Model file for the job. Use its own axes, mm. Face numbers are marked on the shaded views. A direction names the side the tool comes from. Coordinates: 2 decimals unless noted, no trailing zeros. Loops run counter-clockwise (first coordinate to the right, second up) from the corner with the lowest first, then second, coordinate; pieces in that order, holes last.
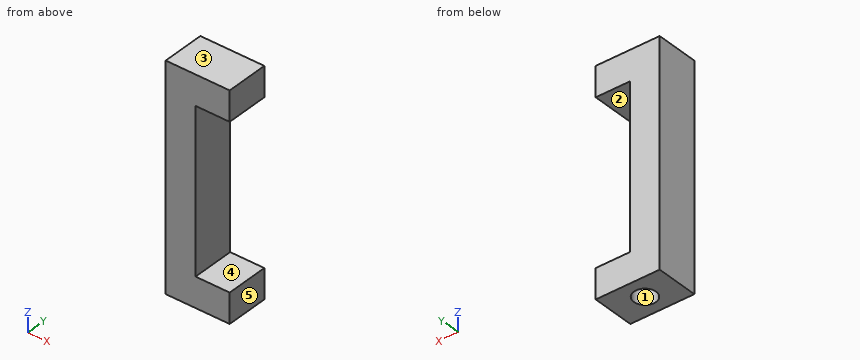
from build123d import *

# Parameters (mm, degrees)
F1_DEPTH      = 12.5
F1_DEPTH_BACK = 12.5
F2_R          = 6.5
F3_DEPTH      = 12


with BuildPart() as f1:
    # F0 (on Front) → F1 (new body, two sides)
    with BuildSketch(Plane.XZ) as f1_sk:
        Polygon((0, 65), (0, 0), (0, -65), (37.5, -65), (37.5, -47.5), (17.5, -47.5), (17.5, 0), (17.5, 47.5), (37.5, 47.5), (37.5, 65), align=None)
    extrude(amount=F1_DEPTH)
    extrude(f1_sk.sketch, amount=-F1_DEPTH_BACK)

    # F2 (on face) → F3 (cut)
    with BuildSketch(Plane(origin=(0, 0, -65), x_dir=(1, 0, 0), z_dir=(0, 0, -1))):
        with Locations((18.75, 0)):
            Circle(F2_R)
    extrude(amount=-F3_DEPTH, mode=Mode.SUBTRACT)


solid = f1.part
Q1. Slice it at A-A (x = 18.75). List the corners of the cut face in (y, z), and give its area (3 significant figures).
Answers:
outline: (-12.5, -65) - (-6.5, -65) - (-6.5, -53) - (6.5, -53) - (6.5, -65) - (12.5, -65) - (12.5, -47.5) - (-12.5, -47.5) - close; (-12.5, 47.5) - (12.5, 47.5) - (12.5, 65) - (-12.5, 65) - close
area: 719 mm2
Q2. Mould opens along Z. For the marked faces 1, 2 and 3 say: +Z half, -Z half, draft (parallel to the pull), parting line (faces both ways), or undercut.
Answers:
face 1: draft
face 2: undercut
face 3: +Z half
Q3. Slice it at C-C (x = 31). List the corners of the cut face in (y, z).
Answers:
outline: (-12.5, -65) - (12.5, -65) - (12.5, -47.5) - (-12.5, -47.5) - close; (-12.5, 47.5) - (12.5, 47.5) - (12.5, 65) - (-12.5, 65) - close
Q4. Slice it at D-D (z = -36.5). List the corners of the cut face in (x, y).
Answers:
outline: (0, -12.5) - (17.5, -12.5) - (17.5, 12.5) - (0, 12.5) - close
Q5. Slice it at B-B (y = 8). List the corners of the cut face in (x, z), and give its area (4 significant figures).
Answers:
outline: (0, -65) - (37.5, -65) - (37.5, -47.5) - (17.5, -47.5) - (17.5, 47.5) - (37.5, 47.5) - (37.5, 65) - (0, 65) - close
area: 2,975 mm2
Q6. Flat gauge pin, fed straight in: P1, Ø2, axis at y = 0, z = 36, coming from the +X side. Where does the tip first touch, or does it go through?
Answers:
P1: stops at x = 17.5
Q7. Which spindle directions (+Z, -Z, +X, -X, +Y, -Y) get a long thin tool onto all of the face, cutting with end or side? Do the marked faces 4 and 5. Say none if no direction does.
Answers:
face 4: +X, +Y, -Y
face 5: +Z, -Z, +X, +Y, -Y
Q8. Drill centre lines: line 1 (X direction, y = 0, z = -57.25); line 2 (Z direction, x = 20, y = 0.75); line 3 (Y direction, x = 18.75, z = -58.5). Where is each one in solid material? Low to high.
Answers:
line 1: x = 0 to 12.25, 25.25 to 37.5
line 2: z = -53 to -47.5, 47.5 to 65
line 3: y = -12.5 to -6.5, 6.5 to 12.5
